Verification items for the finished model (mm, model axes). A direction names the side the tool comes from. Round coordinates to 2 decimals unless told otherwise and drop trailing zeros. Order: outer loops, then holes, each group sorted by start corner. A loop starts at its lowest first (then second) coordinate and runs counter-clockwise, first axis right, second up. Notation, with made-up numbers: M -30,67.25 L 17,67.25 A8 ccw 17,71.25 Z; hole C 18.5,32.5 d4. An arc over 180 degrees is marked long. One line per item, written item: value. Start each with the question number.
from build123d import *

# Parameters (mm, degrees)
SALIENTE_EXTRUIR1_DEPTH = 5
CROQUIS2_R              = 0.5
CORTAR_EXTRUIR1_DEPTH   = 5.67653718
CROQUIS3_R              = 1
CORTAR_EXTRUIR2_DEPTH   = 2


with BuildPart() as part:
    # Croquis1 → Saliente-Extruir1 (new body)
    with BuildSketch(Plane(origin=(0, 0, 0), x_dir=(1, 0, 0), z_dir=(0, 1, 0))):
        Polygon((2.7, 0), (1.35, 2.33826859), (-1.35, 2.33826859), (-2.7, 0), (-1.35, -2.33826859), (1.35, -2.33826859), align=None)
    extrude(amount=SALIENTE_EXTRUIR1_DEPTH)

    # Croquis2 → Cortar-Extruir1 (cut, through all)
    with BuildSketch(Plane.XY.offset(2.33826859)):
        with Locations((0, 1)):
            Circle(CROQUIS2_R)
    extrude(amount=-CORTAR_EXTRUIR1_DEPTH, mode=Mode.SUBTRACT)

    # Croquis3 → Cortar-Extruir2 (cut)
    with BuildSketch(Plane.XY.offset(2.33826859)):
        with Locations((0, 1.5)):
            Circle(CROQUIS3_R)
    extrude(amount=-CORTAR_EXTRUIR2_DEPTH, mode=Mode.SUBTRACT)


solid = part.part
1. Section check D-D (z = 1.2). Record the cut outline in (x, y).
2. Section check A-A (y = 0.7). Record the cut outline in (x, z), and give its area (3 significant figures).
3. Tool access check on faces 1 (the face through (0, 2, -2.338)), 2 (the face through (-0.217, 0.524, 1.352)). Record the directions out of +Z, -Z, +X, -X, +Y, -Y that give a thin tool (end or side, any length) a straight path to the whole face; none if there is none.
4. Section check B-B (z = 0.7). Record the cut outline in (x, y), and give its area (3 significant figures).
5. Section check C-C (y = 3.8). Record the cut outline in (x, z), and give its area (3 significant figures).
6. Draft check along Y on faces 3 (the face through (-0.108, 0.512, -0.981)), 4 (the face through (0, 0, 0)), 5 (the face through (0, 2, 0.338)), 6 (the face through (2.016, 2.465, 1.186)). Enter one of: released by +Y, released by -Y, zero draft, split by the parting line, or undercut.
7. Scan lines: line 1 along Y through (x, z) = (0, -0.95); line 2 along X through (y, z) = (1, -0.55); line 3 along X through (y, z) = (0.8, -0.35). Record each from-to range of solid material in increasing order.
8. Depth check by flat-ended pin: pin 1 (1 mm diameter, centred on x = 2, y = 1.5, fed in from +Z). Enter the tip coordinate at first touch or a pass-through.
Geometry check:
1. outline: M -2.01,0 L 2.01,0 L 2.01,5 L -2.01,5 Z; hole C 0,1.5 d2
2. outline: M -2.7,0 L -1.35,-2.34 L -0.4,-2.34 L -0.4,0.34 L -0.6,0.34 L -0.6,2.34 L -1.35,2.34 Z; M 0.4,-2.34 L 1.35,-2.34 L 2.7,0 L 1.35,2.34 L 0.6,2.34 L 0.6,0.34 L 0.4,0.34 Z
2. area: 14.4 mm²
3. face 1: -Z, +X, -X, +Y, -Y
3. face 2: +Z
4. outline: M -2.3,0 L 2.3,0 L 2.3,5 L -2.3,5 Z; hole C 0,1.5 d2
4. area: 19.8 mm²
5. outline: M -2.7,0 L -1.35,-2.34 L 1.35,-2.34 L 2.7,0 L 1.35,2.34 L -1.35,2.34 Z
5. area: 18.9 mm²
6. face 3: undercut
6. face 4: released by -Y
6. face 5: undercut
6. face 6: zero draft
7. line 1: y = 0 to 0.5, 1.5 to 5
7. line 2: x = -2.38 to -0.5, 0.5 to 2.38
7. line 3: x = -2.5 to -0.46, 0.46 to 2.5
8. pin 1: stops at z = 2.08
